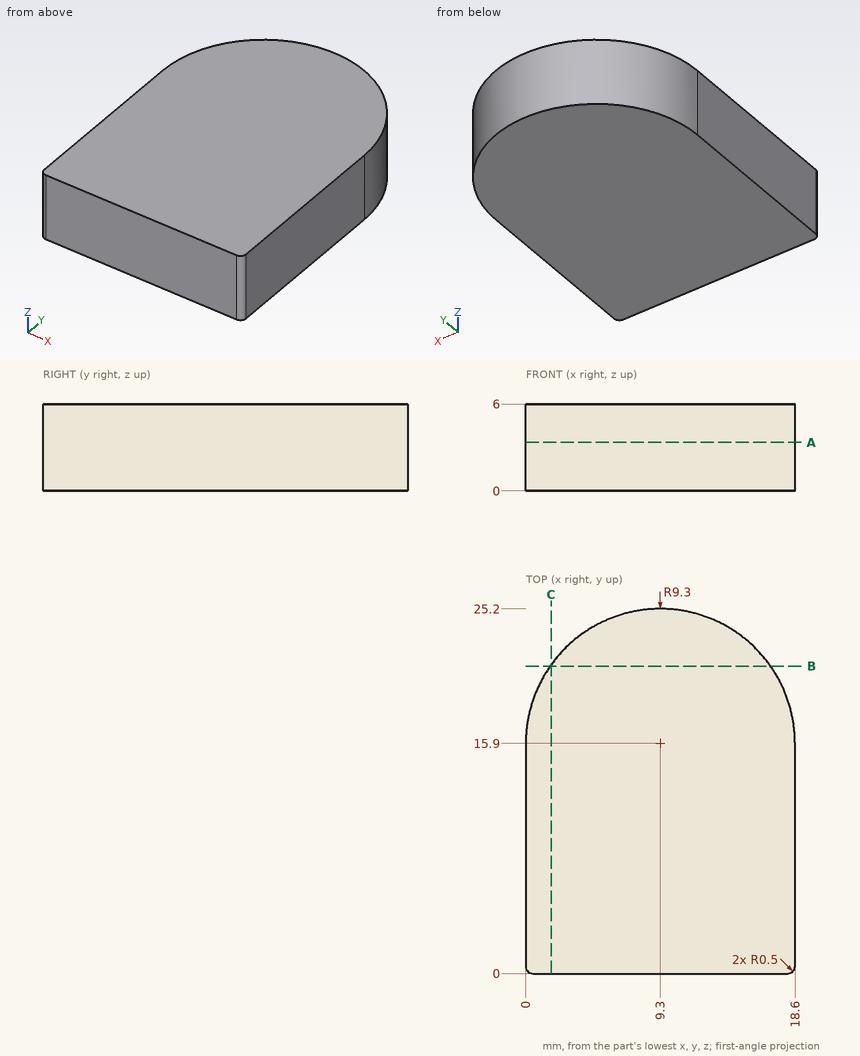
Part print with two shaded views. Sizes in mm from the minimum x, y, z corner. Round coordinates to 2 decimals unless told otherwise and drop trailing zeros. Order: outer loops, then holes, each group sorted by start corner. A loop starts at its lowest first (then second) coordinate and runs counter-clockwise, first axis right, second up. Notation, with made-up numbers: M -4.5,36.5 L 12.5,36.5 A23 ccw 12.5,74.5 Z; hole C -35,-7 d8. An arc over 180 degrees is marked long. Use CSV: the item, a comma, the result in double quotes. Start each with the question number.
(1) Drill centre lines: probe 1 along Y at (x, z) = (12.5, 3.25); probe 2 along Y at (x, z) = (17.75, 4); probe 3 along X at (y, z) = (20, 3.3). Where is each one in solid material? Low to high.
(2) Flat gauge pins, fed straight in: P1, Ø3, axis at x = 6, z = 1, coming from the -Y side; P2, Ø1.5, axis at x = 16.5, z = 3.5, coming from the +Y side. Where does each tip first touch, or does it go through?
(3) Cut at A-A on z = 3.35. List the corners of the cut face in (x, y).
(4) Cut at C-C on x = 1.75. List the corners of the cut face in (y, z).
(5) Cut at B-B on y = 21.25. List the corners of the cut face in (x, z), then the cut area to 3 significant figures.
Findings:
1,probe 1,"y = 0 to 24.63"
1,probe 2,"y = 0 to 19.78"
1,probe 3,"x = 0.95 to 17.65"
2,P1,"stops at y = 0"
2,P2,"stops at y = 22.6"
3,outline,"M 0,0.5 A0.5 ccw 0.5,0 L 18.1,0 A0.5 ccw 18.6,0.5 L 18.6,15.9 A9.3 ccw 0,15.9 Z"
4,outline,"M 0,0 L 21.33,0 L 21.33,6 L 0,6 Z"
5,outline,"M 1.69,0 L 16.91,0 L 16.91,6 L 1.69,6 Z"
5,area,"91.3 mm^2"
